Build history of the part. All positions in model axes, mm. Face numbers are marked on the shaded views. Give positions to 0.01 mm unless a question says otherwise; leave off trailing zeros. Write each loop counter-clockwise with the first axis right and the second up, starting at its lowest first coordinate (ties: lowest second). Pieces come first, ordered by that corner, then holes. Notation, with made-up numbers: M 76.5,77 L 134.5,77 A30 cw 134.5,110 Z; hole C 74.25,29 d1. An arc over 180 degrees is marked long. Return JSON: item names as keys, results as strings. Group by question number.
Q1. Pull direction Y, two halves, no side cores. Call the marked faces 1, 2 and 3: +Y half, -Y half, draft (parallel to the pull), parting line (faces both ways), or undercut.
Q2. Band-saw the part on B-B, the plane y = 6. Count the separate pieces of the cut face and the enclosed holes in it, then the cut area to 3 significant figures.
Q3. Flat gauge pins, fed straight in: pin 1 Ø3 at (x, y) = (18, 3) entering from -Z; pin 2 Ø6 at (x, y) = (-52.95, 6) entering from +Z; pin 3 Ø6.5 at (x, y) = (-78.5, 4.5) entering from +Z. Where does each tip first touch, or does it go through?
Q4. Band-saw the part on A-A, the plane z = -44.5. Give the cut face in (x, y), then the cut area to 3 significant figures.
Q5. Band-saw the part on C-C, the plane x = -34. Give the cut face in (y, z), then the cut area to 3 significant figures.
Q6. Wall check: probe 1 along X at (y, z) = (2.75, -21); probe 2 along X at (y, z) = (6.75, -36); probe 3 along Z at (x, y) = (14.5, 6). Give the ranges that are in metal, low to high.
from build123d import *

# Parameters (mm, degrees)
ESQUISSE1_W             = 180
ESQUISSE1_H             = 18
BOSS_EXTRU_1_DEPTH      = 12
ESQUISSE3_W             = 40
ESQUISSE3_H             = 12
BOSS_EXTRU_2_DEPTH      = 10
ESQUISSE4_R             = 6.05
ENL_V_MAT_EXTRU_1_DEPTH = 12
ENL_V_START             = -28
ESQUISSE5_R             = 2.5
ENL_V_MAT_EXTRU_2_DEPTH = 28
ESQUISSE6_R             = 4
ENL_V_MAT_EXTRU_3_DEPTH = 12
ESQUISSE9_R             = 2.5
ENL_V_MAT_EXTRU_4_DEPTH = 12
CONG_1_R                = 2


with BuildPart() as part:
    # Esquisse1 → Boss.-Extru.1 (new body)
    with BuildSketch(Plane(origin=(0, 0, 0), x_dir=(1, 0, 0), z_dir=(0, 1, 0))):
        with Locations((4.022267576, 28.402118524)):
            Rectangle(ESQUISSE1_W, ESQUISSE1_H)
    extrude(amount=BOSS_EXTRU_1_DEPTH)

    # Esquisse3 → Boss.-Extru.2 (add)
    with BuildSketch(Plane(origin=(0, 0, -37.402118524), x_dir=(-1, 0, 0), z_dir=(0, 0, -1))):
        with Locations((65.977732424, 6)):
            Rectangle(ESQUISSE3_W, ESQUISSE3_H)
    boss_extru_2 = extrude(amount=BOSS_EXTRU_2_DEPTH)

    # Esquisse4 → Enlèv. mat.-Extru.1 (cut)
    with BuildSketch(Plane(origin=(0, 12, 0), x_dir=(1, 0, 0), z_dir=(0, 1, 0))):
        with Locations((-65.977732424, 47.402118524)):
            Circle(ESQUISSE4_R)
    enl_v_mat_extru_1 = extrude(amount=-ENL_V_MAT_EXTRU_1_DEPTH, mode=Mode.SUBTRACT)

    # Esquisse5 → Enlèv. mat.-Extru.2 (cut)
    with BuildSketch(Plane(origin=(0, 0, -47.402118524), x_dir=(-1, 0, 0), z_dir=(0, 0, -1)).offset(ENL_V_START)):
        with Locations((52.952732424, 6)):
            Circle(ESQUISSE5_R)
        with Locations((79.002732424, 6)):
            Circle(ESQUISSE5_R)
    enl_v_mat_extru_2 = extrude(amount=ENL_V_MAT_EXTRU_2_DEPTH, mode=Mode.SUBTRACT)

    # Esquisse6 → Enlèv. mat.-Extru.3 (cut)
    with BuildSketch(Plane.XY.offset(-19.402118524)):
        with Locations((-52.952732424, 6)):
            Circle(ESQUISSE6_R)
        with Locations((-79.002732424, 6)):
            Circle(ESQUISSE6_R)
    extrude(amount=-ENL_V_MAT_EXTRU_3_DEPTH, mode=Mode.SUBTRACT)

    # Symétrie4: Boss.-Extru.2, Enlèv. mat.-Extru.1, Enlèv. mat.-Extru.2 across plane
    add(boss_extru_2.mirror(Plane(origin=(4.022267576, 12, -19.402118524), x_dir=(0, 0, 1), z_dir=(-1, 0, 0))))
    add(enl_v_mat_extru_1.mirror(Plane(origin=(4.022267576, 12, -19.402118524), x_dir=(0, 0, 1), z_dir=(-1, 0, 0))), mode=Mode.SUBTRACT)
    add(enl_v_mat_extru_2.mirror(Plane(origin=(4.022267576, 12, -19.402118524), x_dir=(0, 0, 1), z_dir=(-1, 0, 0))), mode=Mode.SUBTRACT)

    # Esquisse9 → Enlèv. mat.-Extru.4 (cut)
    with BuildSketch(Plane(origin=(0, 12, 0), x_dir=(1, 0, 0), z_dir=(0, 1, 0))):
        with Locations(Location((4.022267576, 28.402118524, 0), (0, 0, 270))):
            Circle(ESQUISSE9_R)
        with Locations(Location((74.022267576, 28.402118524, 0), (0, 0, 270))):
            Circle(ESQUISSE9_R)
        with Locations(Location((-65.977732424, 28.402118524, 0), (0, 0, 270))):
            Circle(ESQUISSE9_R)
    extrude(amount=-ENL_V_MAT_EXTRU_4_DEPTH, mode=Mode.SUBTRACT)

    # Congé1
    cong_1_edges = [part.edges().sort_by_distance(p)[0] for p in [
        (94.022267576, 12, -33.402118524),
        (-45.977732424, 6, -37.402118524),
        (-45.977732424, 12, -42.402118524),
        (-85.977732424, 12, -33.402118524),
        (4.022267576, 12, -37.402118524),
        (54.022267576, 12, -42.402118524),
        (54.022267576, 6, -37.402118524),
        (94.022267576, 6, -19.402118524),
        (-85.977732424, 6, -19.402118524),
    ]]
    fillet(cong_1_edges, radius=CONG_1_R)


solid = part.part
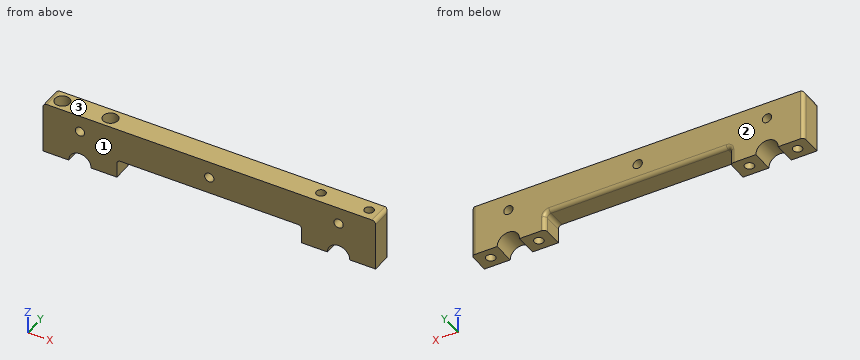
From the geometry:
{
 "1": {"face 1": "-Y half", "face 2": "+Y half", "face 3": "draft"},
 "2": {"separate pieces": "5", "enclosed holes": "3", "area": "3,230 mm^2"},
 "3": {"pin 1": "stops at z = -37.4", "pin 2": "stops at z = -31.4", "pin 3": "stops at z = -19.4"},
 "4": {"outline": "M -85.98,0 L -71.29,0 L -71.29,12 L -83.98,12 A2 ccw -85.98,10 Z; M -60.67,0 L -45.98,0 L -45.98,10 A2 ccw -47.98,12 L -60.67,12 Z; M 54.02,0 L 68.71,0 L 68.71,12 L 56.02,12 A2 ccw 54.02,10 Z; M 79.33,0 L 94.02,0 L 94.02,10 A2 ccw 92.02,12 L 79.33,12 Z; hole C -79,6 d5; hole C -52.95,6 d5; hole C 61,6 d5; hole C 87.05,6 d5", "area": "623 mm^2"},
 "5": {"outline": "M 0,-37.4 L 10,-37.4 A2 ccw 12,-35.4 L 12,-19.4 L 0,-19.4 Z", "area": "215 mm^2"},
 "6": {"probe 1": "x = -85.94 to -81.33, -76.67 to -55.28, -50.62 to 93.98", "probe 2": "x = -85.98 to -81.39, -76.62 to -55.34, -50.57 to 58.61, 63.38 to 84.66, 89.43 to 94.02", "probe 3": "z = -37.4 to -19.4"}
}
